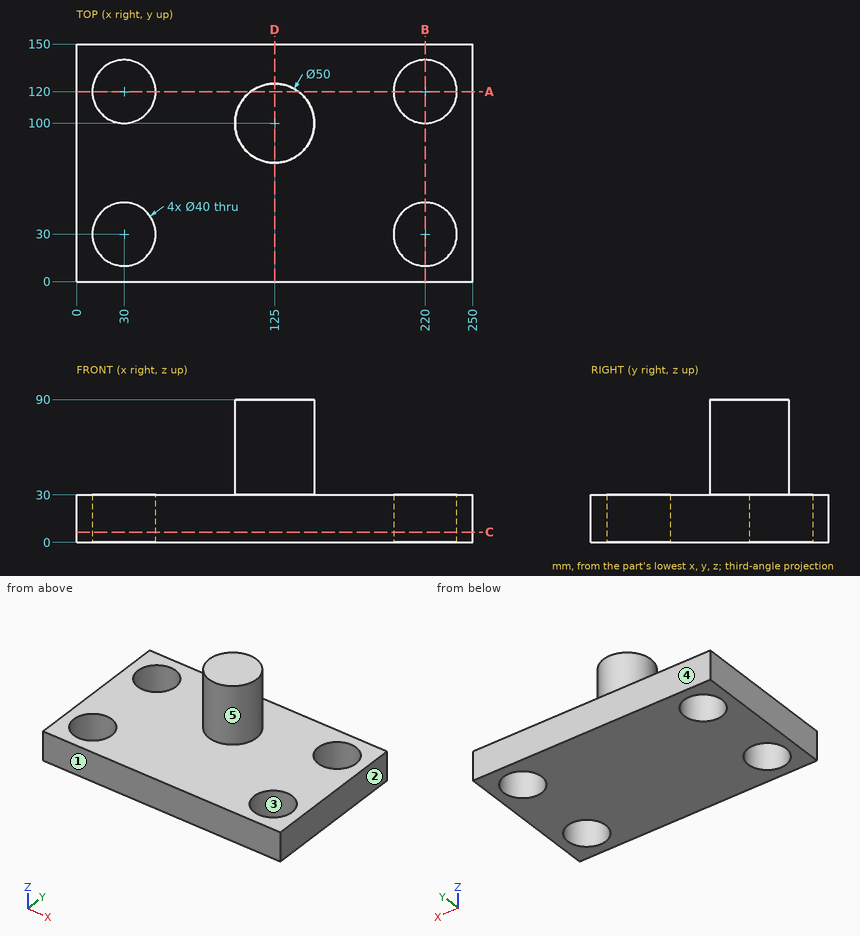
Part print with two shaded views. Sizes in mm from the minimum x, y, z corner. A direction names the side the tool comes from. Round coordinates to 2 decimals unless told otherwise and drop trailing zeros. Order: outer loops, then holes, each group sorted by start corner. A loop starts at its lowest first (then second) coordinate and runs counter-clockwise, first axis right, second up. Notation, with made-up numbers: (45, 52) - (78, 52) arc R28 ccw to (78, 77) - close; hole circle Ø9 at (-19, 79.5). An arc over 180 degrees is marked (long way). Return JSON: item names as keys, results as strings.
(1) Cut at D-D (x = 125). Give the cut face in (y, z).
Answer key:
{"outline": "(0, 0) - (150, 0) - (150, 30) - (125, 30) - (125, 90) - (75, 90) - (75, 30) - (0, 30) - close"}
(2) Tool access for the marked faces 4 and 5: list every direction of +Z, -Z, +X, -X, +Y, -Y with a clear straight run to the whole face (end or side of a thin tool).
Answer key:
{"face 4": "+Z, -Z, +X, -X, +Y", "face 5": "+Z"}
(3) Cut at A-A (y = 120). Give the cut face in (x, z).
Answer key:
{"outline": "(0, 0) - (10, 0) - (10, 30) - (0, 30) - close; (50, 0) - (200, 0) - (200, 30) - (140, 30) - (140, 90) - (110, 90) - (110, 30) - (50, 30) - close; (240, 0) - (250, 0) - (250, 30) - (240, 30) - close"}
(4) Cut at C-C (z = 6.5). Give the cut face in (x, y).
Answer key:
{"outline": "(0, 0) - (250, 0) - (250, 150) - (0, 150) - close; hole circle Ø40 at (30, 30); hole circle Ø40 at (30, 120); hole circle Ø40 at (220, 30); hole circle Ø40 at (220, 120)"}
(5) Cut at B-B (x = 220). Give the cut face in (y, z), then the cut area to 3 significant figures.
Answer key:
{"outline": "(0, 0) - (10, 0) - (10, 30) - (0, 30) - close; (50, 0) - (100, 0) - (100, 30) - (50, 30) - close; (140, 0) - (150, 0) - (150, 30) - (140, 30) - close", "area": "2,100 mm^2"}
(6) Wall check: probe 1 along Y at (x, z) = (220, 22.75); probe 2 along Y at (x, z) = (202, 21.5); probe 3 along Z at (x, y) = (33, 99). Give the ranges that are in metal, low to high. Write a range as from..to.
Answer key:
{"probe 1": "y = 0..10, 50..100, 140..150", "probe 2": "y = 0..21.28, 38.72..111.28, 128.72..150", "probe 3": "z = 0..30"}
(7) Pin check, flat tips, straight feed: pin 1 Ø1.5 at (x, y) = (146.5, 82.5) entering from +Z; pin 2 Ø2 at (x, z) = (92.5, 12) entering from -Y. Stop position of each tip, or through.
Answer key:
{"pin 1": "stops at z = 30", "pin 2": "stops at y = 0"}
(8) Pull direction X, two halves, no side cores. Call the marked faces 1, 2 and 3: +X half, -X half, draft (parallel to the pull), parting line (faces both ways), or undercut.
Answer key:
{"face 1": "draft", "face 2": "+X half", "face 3": "undercut"}
